Build history of the part. All positions in model axes, mm. A direction names the side the tool comes from. Give positions to 0.01 mm unless a question says otherwise; leave off trailing zeros. Write each loop counter-clockwise with the first axis right and the second up, starting at its lowest first coordinate (ties: lowest second). Pieces come first, ordered by that corner, then holes. Notation, with made-up numbers: (-35, 57) -> (-16, 57) arc R33 ccw to (-16, 89) -> close; hole circle Ø4 at (-10, -5). An arc over 180 degrees is marked (long way). One line per question, with ' | ' between items. Start each with the question number.
(1) Band-saw the part on A-A, the plane z = 16.5. Give the cut face in (x, y).
(2) Band-saw the part on C-C, the plane z = 5. Give the cut face in (x, y).
(3) Drill centre lines: probe 1 along Y at (x, z) = (16.25, 5); probe 2 along Y at (x, z) = (105.9, 15); probe 3 along X at (y, z) = (29, 2.75). Where is each one in solid material? Low to high. Write a range as from..to.
(4) Tool access for faces 5 (the flat face through (150, -1, 5)), 6 (the cylindrical face through (49.517, -0.17, 15.563)), 7 (the flat face through (30, 0, 5)): list every direction of +Z, -Z, +X, -X, +Y, -Y with a clear straight run to the whole face (end or side of a thin tool).
(5) Band-saw the part on D-D, the plane x = 105.9. Give the cut face in (y, z).
(6) Pin check, flat tips, straight feed: P1, Ø1, axis at y = -2, z = 2.5, coming from the -X side; P2, Ø3, axis at x = 48, y = 0.5, coming from the +Z side; P3, Ø1.5, axis at x = 82, y = -2.5, coming from the +Z side. Stop position of each tip, or through.
(7) Band-saw the part on B-B, the plane y = -48.5. Give the cut face in (x, z).
(8) Pull direction Y, two halves, no side cores. Call faces 1 (the flat face through (74, -60, 5)), 2 (the cylindrical face through (103.4, 0.7, 14.9)), 3 (the flat face through (74, 1, 0)), 4 (the flat face through (74, 60, 5)): released by +Y, released by -Y, zero draft, split by the parting line, or undercut.
from build123d import *

# Parameters (mm, degrees)
SKETCH1_W               = 150
SKETCH1_H               = 120
BOSS_EXTRUDE1_DEPTH     = 10
SKETCH2_R               = 4
CUT_EXTRUDE1_DEPTH      = 30
CROQUIS4_R              = 2.5
SALIENTE_EXTRUIR2_DEPTH = 10
CROQUIS5_R              = 1.75
CORTAR_EXTRUIR1_DEPTH   = 9


with BuildPart() as part:
    # Sketch1 → Boss-Extrude1 (new body)
    with BuildSketch(Plane.XY):
        with Locations((75, 0)):
            Rectangle(SKETCH1_W, SKETCH1_H)
    extrude(amount=BOSS_EXTRUDE1_DEPTH)

    # Sketch2 → Cut-Extrude1 (cut)
    with BuildSketch(Plane.ZY):
        with Locations((5, 0)):
            Circle(SKETCH2_R)
        with Locations((5, 30)):
            Circle(SKETCH2_R)
        with Locations((5, -30)):
            Circle(SKETCH2_R)
    extrude(amount=-CUT_EXTRUDE1_DEPTH, mode=Mode.SUBTRACT)

    # Croquis4 → Saliente-Extruir2 (add)
    with BuildSketch(Plane.XY.offset(10)):
        with Locations((47.900115216, 0.5)):
            Circle(CROQUIS4_R)
        with Locations((105.9, 0.615607451)):
            Circle(CROQUIS4_R)
        with Locations((105.9, -48.5)):
            Circle(CROQUIS4_R)
        with Locations((47.900115216, -48.5)):
            Circle(CROQUIS4_R)
    extrude(amount=SALIENTE_EXTRUIR2_DEPTH)

    # Croquis5 → Cortar-Extruir1 (cut)
    with BuildSketch(Plane.XY.offset(20)):
        with Locations((47.900115216, 0.5)):
            Circle(CROQUIS5_R)
        with Locations((47.900115216, -48.5)):
            Circle(CROQUIS5_R)
        with Locations((105.9, -48.5)):
            Circle(CROQUIS5_R)
        with Locations((105.9, 0.615607451)):
            Circle(CROQUIS5_R)
    extrude(amount=-CORTAR_EXTRUIR1_DEPTH, mode=Mode.SUBTRACT)


solid = part.part
Results:
1) outline: circle Ø5 at (47.9, -48.5); circle Ø5 at (47.9, 0.5); circle Ø5 at (105.9, -48.5); circle Ø5 at (105.9, 0.62); hole circle Ø3.5 at (47.9, -48.5); hole circle Ø3.5 at (47.9, 0.5); hole circle Ø3.5 at (105.9, -48.5); hole circle Ø3.5 at (105.9, 0.62)
2) outline: (0, -60) -> (150, -60) -> (150, 60) -> (0, 60) -> (0, 34) -> (30, 34) -> (30, 26) -> (0, 26) -> (0, 4) -> (30, 4) -> (30, -4) -> (0, -4) -> (0, -26) -> (30, -26) -> (30, -34) -> (0, -34) -> close
3) probe 1: y = -60..-34, -26..-4, 4..26, 34..60 | probe 2: y = -51..-50.25, -46.75..-46, -1.88..-1.13, 2.37..3.12 | probe 3: x = 30..150
4) face 5: +Z, -Z, +X, +Y, -Y | face 6: +Z | face 7: -X
5) outline: (-60, 0) -> (60, 0) -> (60, 10) -> (3.12, 10) -> (3.12, 20) -> (2.37, 20) -> (2.37, 11) -> (-1.13, 11) -> (-1.13, 20) -> (-1.88, 20) -> (-1.88, 10) -> (-46, 10) -> (-46, 20) -> (-46.75, 20) -> (-46.75, 11) -> (-50.25, 11) -> (-50.25, 20) -> (-51, 20) -> (-51, 10) -> (-60, 10) -> close
6) P1: stops at x = 30 | P2: stops at z = 11 | P3: stops at z = 10
7) outline: (0, 0) -> (150, 0) -> (150, 10) -> (108.4, 10) -> (108.4, 20) -> (107.65, 20) -> (107.65, 11) -> (104.15, 11) -> (104.15, 20) -> (103.4, 20) -> (103.4, 10) -> (50.4, 10) -> (50.4, 20) -> (49.65, 20) -> (49.65, 11) -> (46.15, 11) -> (46.15, 20) -> (45.4, 20) -> (45.4, 10) -> (0, 10) -> close
8) face 1: released by -Y | face 2: undercut | face 3: zero draft | face 4: released by +Y
